Source: CAD feature listing. Evaluate the final solid. Frame: model axes, mm. A direction names the side the tool comes from. Round coordinates to 2 decimals unless told otherwise and drop trailing zeros. One line per item, written item: value. Start each with the question number.
1) Ray query, L1, parallel to Z at x = 45, y = -62. Return the intervals inside material, ascending.
2) Mould query, pull axis X, two halves, no side actions, for faces 3 (the face through (75, -1, 42)), 4 (the face through (-69, -60, 16)), 5 (the face through (-1, 70, 42)). Classes: pulls with the +X half, pulls with the -X half, needs draft (parallel to the pull), parting line crosses it, or undercut.
3) Pin query (flat end, axial travel): P1, Ø5, axis at x = -69, z = 81, coming from the -Y side; P2, Ø1.4, axis at x = -69, z = 16.5, coming from the -Y side. Return the tip coordinate at first contact, or that it passes through.
4) Reachability of faces 1 (the face through (-70.755, -65.07, 17.609)), 2 (the face through (-1, 1, 86)) from +Z, -Z, +X, -X, +Y, -Y: full face, straight path, thin tool, end or side. Return the list, or none.
```python
from build123d import *

# Parameters (mm, degrees)
F0_W     = 150
F0_H     = 140
F1_DEPTH = 86
F2_R     = 2.38125
F3_DEPTH = 10


with BuildPart() as f1:
    # F0 (on Top) → F1 (new body)
    with BuildSketch(Plane.XY):
        Rectangle(F0_W, F0_H)
    extrude(amount=F1_DEPTH)

    # F2 (on face) → F3 (cut)
    with BuildSketch(Plane.XZ.offset(70)):
        with Locations((-69, 80)):
            Circle(F2_R)
        with Locations((-69, 16)):
            Circle(F2_R)
        with Locations((69, 80)):
            Circle(F2_R)
        with Locations((45, 6)):
            Circle(F2_R)
    extrude(amount=-F3_DEPTH, mode=Mode.SUBTRACT)


solid = f1.part
```
Findings:
1. L1: 0 to 3.62, 8.38 to 86
2. face 3: pulls with the +X half
2. face 4: undercut
2. face 5: needs draft
3. P1: y = -70
3. P2: y = -60
4. face 1: -Y
4. face 2: +Z, +X, -X, +Y, -Y
